Build history of the part. All positions in model axes, mm. Face numbers are marked on the shaded views. Give positions to 0.01 mm unless a question says otherwise; leave off trailing zeros. Write each loop counter-clockwise with the first axis right and the second up, starting at its lowest first coordinate (ties: lowest second). Pieces come first, ordered by that corner, then holes. Notation, with made-up numbers: (80.25, 54.5) -> (112.25, 54.5) arc R26 ccw to (112.25, 70.5) -> close; hole circle Ø2 at (12, 71.25). An arc over 180 degrees is marked (long way). Put each result on its own line as item: value. Start each with the question number.
Item 1: Flat gauge pins, fed straight in: pin 1 Ø1 at (x, z) = (-1, -1) entering from +Y; pin 2 Ø1 at (x, y) = (-9.5, -4.5) entering from -Z; pin 3 Ø1 at (x, z) = (3.5, 0) entering from +Y. Where does each tip first touch, or does it go through?
Item 2: Two-plate mould, pull along Y, no slides. Class the marked faces 1, 2 and 3: pulls with the +Y half, pulls with the -Y half, needs draft (parallel to the pull), parting line crosses it, or undercut.
Item 3: Slice it at A-A, the plane x = 0. List the corners of the cut face in (y, z).
Item 4: Drill centre lines: line 1 along Y through (x, z) = (0, -0.65); line 2 along Y through (x, z) = (1.5, -0.7); line 3 along X through (y, z) = (-0.5, -0.5). Where is each one in solid material? Low to high.
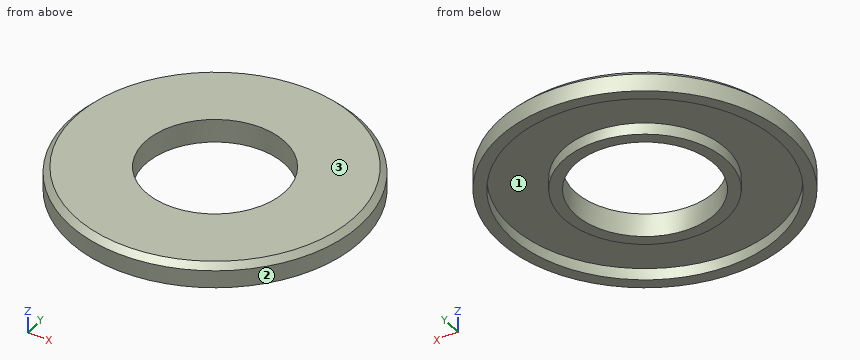
```python
from build123d import *

# Parameters (mm, degrees)
F0_R     = 12.5
F0_R_2   = 11.5
F0_R_3   = 7
F0_R_4   = 6
F1_DEPTH = 1
F2_DEPTH = 1
F3_SIZE  = 0.5


with BuildPart() as f1:
    # F0 (on Top) → F1 (new body)
    with BuildSketch(Plane.XY):
        Circle(F0_R)
        Circle(F0_R_2, mode=Mode.SUBTRACT)
        Circle(F0_R_2)
        Circle(F0_R_3, mode=Mode.SUBTRACT)
        Circle(F0_R_3)
        Circle(F0_R_4, mode=Mode.SUBTRACT)
    extrude(amount=F1_DEPTH)

    # F0 (on Top) → F2 (join)
    with BuildSketch(Plane.XY):
        Circle(F0_R)
        Circle(F0_R_2, mode=Mode.SUBTRACT)
        Circle(F0_R_3)
        Circle(F0_R_4, mode=Mode.SUBTRACT)
    extrude(amount=-F2_DEPTH)

    # F3
    f3_edges = [f1.edges().sort_by_distance(p)[0] for p in [
        (-12.5, 0, 1),
    ]]
    chamfer(f3_edges, length=F3_SIZE)


solid = f1.part
```
Values follow:
1. pin 1: y = 12.49
1. pin 2: z = 0
1. pin 3: y = 12.13
2. face 1: undercut
2. face 2: parting line crosses it
2. face 3: needs draft
3. outline: (-12.5, -1) -> (-11.5, -1) -> (-11.5, 0) -> (-7, 0) -> (-7, -1) -> (-6, -1) -> (-6, 1) -> (-12, 1) -> (-12.5, 0.5) -> close; (6, -1) -> (7, -1) -> (7, 0) -> (11.5, 0) -> (11.5, -1) -> (12.5, -1) -> (12.5, 0.5) -> (12, 1) -> (6, 1) -> close
4. line 1: -12.5 to -11.5, -7 to -6, 6 to 7, 11.5 to 12.5
4. line 2: -12.41 to -11.4, -6.84 to -5.81, 5.81 to 6.84, 11.4 to 12.41
4. line 3: -12.49 to -11.49, -6.98 to -5.98, 5.98 to 6.98, 11.49 to 12.49
